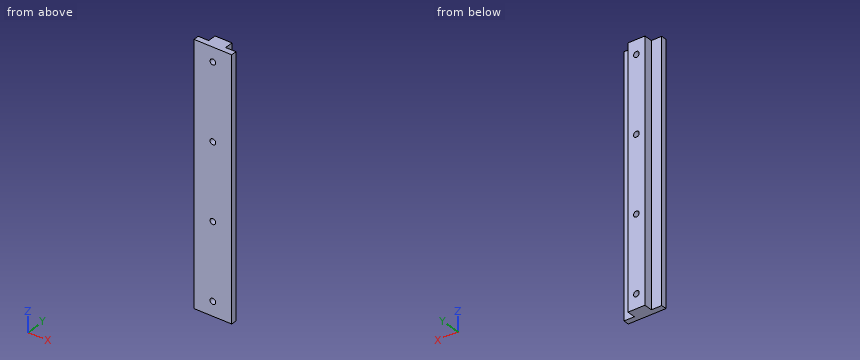
Autodesk Inventor part; units mm, degrees
ref_plane "YZ Plane" through (0, 0, 0) normal (1, 0, 0) x (0, 1, 0)
ref_plane "XZ Plane" through (0, 0, 0) normal (0, 1, 0) x (-1, 0, 0)
ref_plane "XY Plane" through (0, 0, 0) normal (0, 0, 1) x (1, 0, 0)
sketch "スケッチ1" plane through (0, 0, 0) normal (0, 0, 1) x (1, 0, 0)
  line L0 (-10, 3) -> (-4.5, 3)
  line L1 (10, 3) -> (10, 0)
  line L2 (10, 0) -> (-10, 0)
  line L3 (-10, 0) -> (-10, 3)
  line L4 (-10, 3) -> (10, 0) construction
  line L5 (10, 3) -> (-10, 0) construction
  line L6 (-4.5, 7.5) -> (4.5, 7.5)
  line L7 (4.5, 7.5) -> (4.5, 3)
  line L8 (-4.5, 3) -> (-4.5, 7.5)
  line L9 (-4.5, 7.5) -> (4.5, 3) construction
  line L10 (4.5, 7.5) -> (-4.5, 3) construction
  line L11 (4.5, 3) -> (10, 3)
  point P0 (0, 0)
  point P1 (0, 1.5)
  point P2 (0, 5.25)
  dimension "d0" = 20
  dimension "d1" = 3
  dimension "d2" = 9
  dimension "d3" = 4.5
extrude "押し出し1" add sketch "スケッチ1" along normal blind 135
sketch "スケッチ2" plane through (-4.5, 7.5, 0) normal (0, 1, 0) x (1, 0, 0)
  line L0 (0, 0) -> (9, 0)
  line L1 (9, -135) -> (0, -135)
  point P0 (4.5, 0)
  point P1 (4.5, -7.5)
  point P2 (4.5, -47.5)
  point P3 (4.5, -87.5)
  point P4 (4.5, -127.5)
  dimension "d6" = 7.5
  dimension "d7" = 40
  dimension "d8" = 40
  dimension "d9" = 40
  dimension "d10" = 7.5
hole "穴1" at (0, 7.5, 7.5) at (0, 7.5, 47.5) at (0, 7.5, 87.5) at (0, 7.5, 127.5) direction (0, -1, 0) diameter 3 end through all
properties part number "slider_b7p5x20_135_sa" material "アルミニウム 6061-AHC"
The model under review builds one solid part; all positions refer to its coordinate system, in mm. Round coordinates to 2 decimals unless told otherwise and drop trailing zeros. Write each loop counter-clockwise with the first axis right and the second up, starting at its lowest first coordinate (ties: lowest second). Pieces come first, ordered by that corner, then holes.
(1) Insertion check: pin 1 (3 mm diameter, centred on x = -7, z = 89, fed in from +Y); pin 2 (1.3 mm diameter, centred on y = 6, z = 47, fed in from -X); pin 3 (1.3 mm diameter, centred on y = 6, z = 89, fed in from +X). Each pin has a flat end and moves straight along its axis. Give the tip position at first contact, or say it passes through.
(2) We need section A-A on x = 0. Give the boundary of the cut face in (y, z).
(3) We need section B-B on z = 7.5. Give the boundary of the cut face in (x, y).
(4) We need section D-D on z = 103. Give the boundary of the cut face in (x, y).
(5) We need section C-C on y = 5. Give the boundary of the cut face in (x, z), and give its area (3 significant figures).
(6) Wall thickness on L1, parallel to Z at x = 0, y = 2.5; L2, parallel to X at y = 5.5, z = 47.5; L3, parallel to Y at x = 5.75, z = 64: over which ranges is each line inside the solid? List them lowest first.
Findings below:
1. pin 1: stops at y = 3
1. pin 2: stops at x = -4.5
1. pin 3: stops at x = 4.5
2. outline: (0, 0) - (7.5, 0) - (7.5, 6) - (0, 6) - close; (0, 9) - (7.5, 9) - (7.5, 46) - (0, 46) - close; (0, 49) - (7.5, 49) - (7.5, 86) - (0, 86) - close; (0, 89) - (7.5, 89) - (7.5, 126) - (0, 126) - close; (0, 129) - (7.5, 129) - (7.5, 135) - (0, 135) - close
3. outline: (-10, 0) - (-1.5, 0) - (-1.5, 7.5) - (-4.5, 7.5) - (-4.5, 3) - (-10, 3) - close; (1.5, 0) - (10, 0) - (10, 3) - (4.5, 3) - (4.5, 7.5) - (1.5, 7.5) - close
4. outline: (-10, 0) - (10, 0) - (10, 3) - (4.5, 3) - (4.5, 7.5) - (-4.5, 7.5) - (-4.5, 3) - (-10, 3) - close
5. outline: (-4.5, 0) - (4.5, 0) - (4.5, 135) - (-4.5, 135) - close; hole circle Ø3 at (0, 7.5); hole circle Ø3 at (0, 47.5); hole circle Ø3 at (0, 87.5); hole circle Ø3 at (0, 127.5)
5. area: 1,190 mm2
6. L1: z = 0 to 6, 9 to 46, 49 to 86, 89 to 126, 129 to 135
6. L2: x = -4.5 to -1.5, 1.5 to 4.5
6. L3: y = 0 to 3
